Check sheet for the drawn part. Datum: minimum x, y, z corner. Units: mm. Round coordinates to 2 decimals unless told otherwise and drop trailing zeros. Order: outer loops, then holes, each group sorted by start corner. A loop starts at its lowest first (then second) coordinate and runs counter-clockwise, first axis right, second up. Notation, with made-up numbers: (74.5, 52.25) - (131.5, 52.25) arc R34 ccw to (131.5, 89.25) - close; hole circle Ø9 at (-22.5, -22.75). An arc over 180 degrees is marked (long way). Write each question's results on one line, items separated by ' | '.
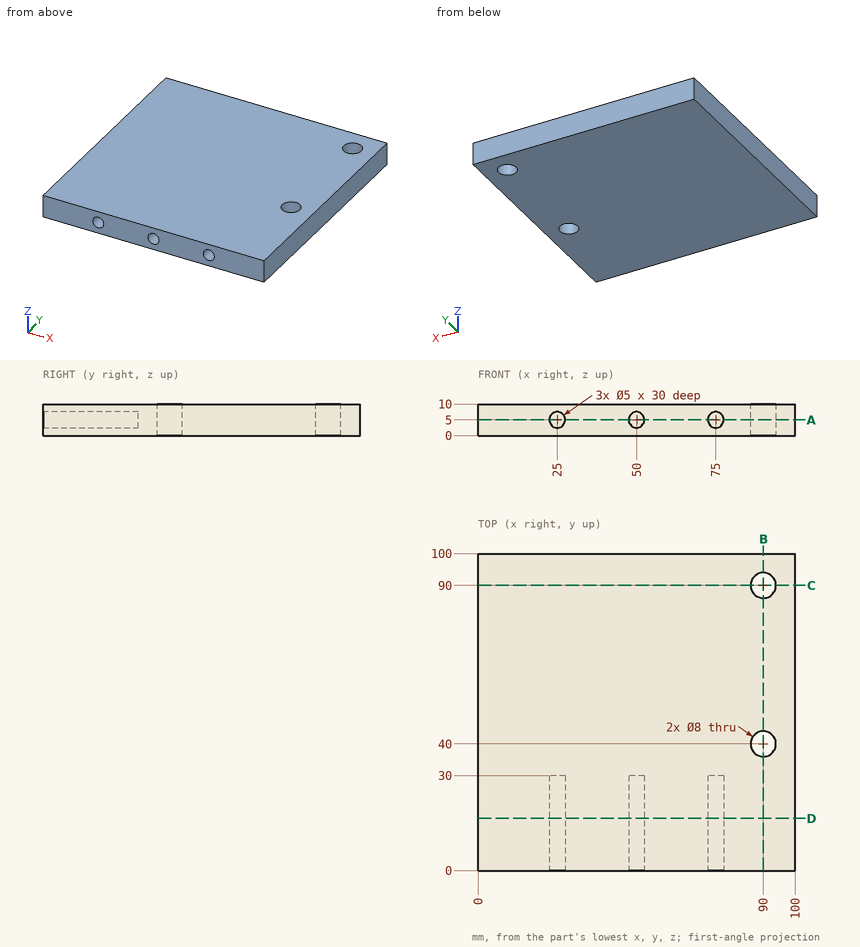
(1) Section check C-C (y = 90). Record the cut outline in (x, z).
Answers follow:
outline: (0, 0) - (86, 0) - (86, 10) - (0, 10) - close; (94, 0) - (100, 0) - (100, 10) - (94, 10) - close
(2) Section check D-D (y = 16.5). Record the cut outline in (x, z), then the cut area to 3 significant figures.
Answers follow:
outline: (0, 0) - (100, 0) - (100, 10) - (0, 10) - close; hole circle Ø5 at (25, 5); hole circle Ø5 at (50, 5); hole circle Ø5 at (75, 5) | area: 941 mm²
(3) Material ranges on line 1 (Y direction, x = 90, z = 7.25); line 2 (X direction, y = 15.75, z = 5); line 3 (X direction, y = 19, z = 6), recorded low to high.
Answers follow:
line 1: 0 to 36, 44 to 86, 94 to 100 | line 2: 0 to 22.5, 27.5 to 47.5, 52.5 to 72.5, 77.5 to 100 | line 3: 0 to 22.71, 27.29 to 47.71, 52.29 to 72.71, 77.29 to 100
(4) Section check A-A (z = 5). Record the cut outline in (x, y).
Answers follow:
outline: (0, 0) - (22.5, 0) - (22.5, 30) - (27.5, 30) - (27.5, 0) - (47.5, 0) - (47.5, 30) - (52.5, 30) - (52.5, 0) - (72.5, 0) - (72.5, 30) - (77.5, 30) - (77.5, 0) - (100, 0) - (100, 100) - (0, 100) - close; hole circle Ø8 at (90, 40); hole circle Ø8 at (90, 90)
(5) Section check B-B (x = 90). Record the cut outline in (y, z), then the cut area to 3 significant figures.
Answers follow:
outline: (0, 0) - (36, 0) - (36, 10) - (0, 10) - close; (44, 0) - (86, 0) - (86, 10) - (44, 10) - close; (94, 0) - (100, 0) - (100, 10) - (94, 10) - close | area: 840 mm²
(6) Depth check by flat-ended pin: pin 1 Ø1.5 at (x, z) = (51, 5) entering from -Y. Enter the tip coordinate at first touch or a pass-through.
Answers follow:
pin 1: y = 30
